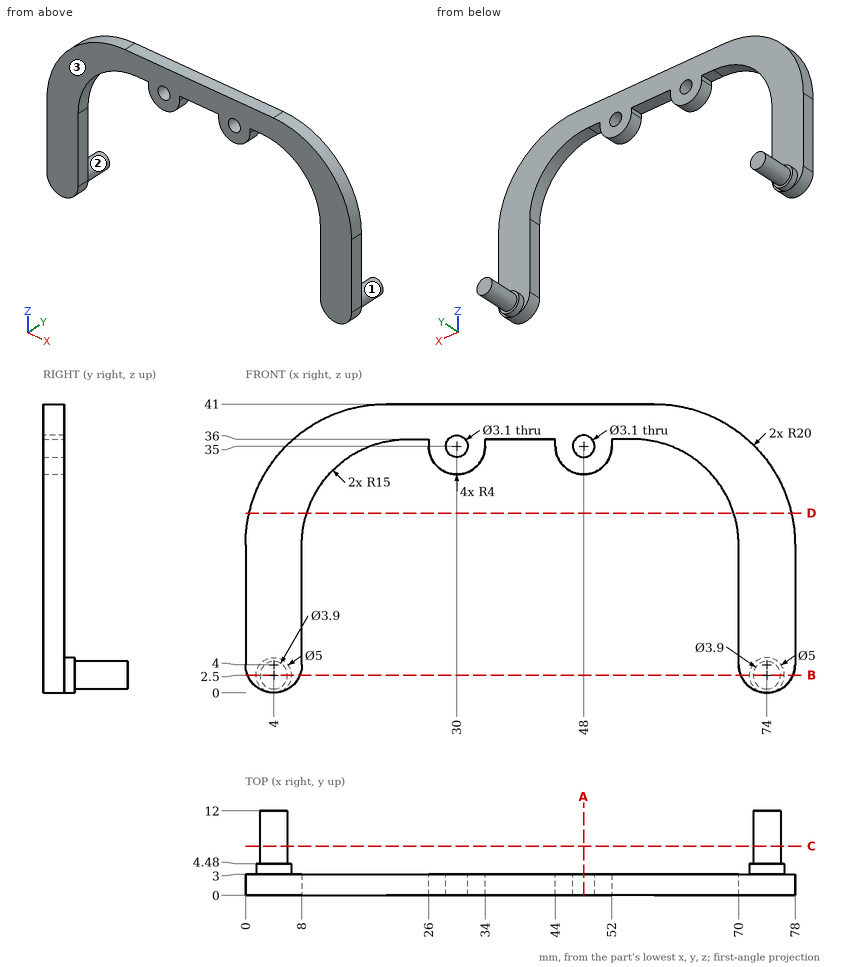
Can you work these out from the drawing? Everything is in mm from the part's minimum corner. Give positions to 0.01 mm unless a question says otherwise; leave off trailing zeros. Loops run counter-clockwise (first coordinate to the right, second up) from the corner with the lowest first, then second, coordinate; pieces in that order, holes last. Notation, with made-up numbers: (25.25, 59.5) - (34.25, 59.5) arc R24 cw to (34.25, 87.5) - close; hole circle Ø10 at (22, 47). An arc over 180 degrees is marked (long way). Use one line per item in the form item = value.
1. I want a section at D-D (z = 25.5). Please give me the cut outline in (x, y), and give its area (3 significant figures).
Response values:
outline = (0.51, 0) - (8.69, 0) - (8.69, 3) - (0.51, 3) - close; (69.31, 0) - (77.49, 0) - (77.49, 3) - (69.31, 3) - close
area = 49.1 mm²
2. I want a section at C-C (y = 7). Please give me the cut outline in (x, z), and give its area (3 significant figures).
Response values:
outline = circle Ø3.9 at (4, 2.5); circle Ø3.9 at (74, 2.5)
area = 23.9 mm²
3. I'm going to push flat-ended pins straight in: pin 1 Ø20.5 at (x, z) = (58, 28.5) entering from +Y; pin 2 Ø1.9 at (x, z) = (48, 35) entering from -Y; pin 3 Ø0.5 at (y, z) = (2, 35.5) entering from -X; pin 4 Ø0.8 at (y, z) = (1.5, 35.5) entering from +X. Where does each tip first touch, or does it pass through?
Response values:
pin_1 = 3
pin_2 = through
pin_3 = 5.97
pin_4 = 72.18
4. I need wall thicknesses on probe 1 along Z at (x, y) = (48, 1.35); probe 2 along Y at (x, z) = (59.5, 39); probe 3 along Z at (x, y) = (68, 2). Which ranges of each line are inside material? Lowest first, please.
Response values:
probe_1 = 31 to 33.45, 36.55 to 41
probe_2 = 0 to 3
probe_3 = 28.48 to 38.32
5. I want a section at A-A (x = 48). Please give me the cut outline in (y, z).
Response values:
outline = (0, 31) - (3, 31) - (3, 33.45) - (0, 33.45) - close; (0, 36.55) - (3, 36.55) - (3, 41) - (0, 41) - close
6. Thinking about a two-plate mould opening in X: for the marked faces 1, 2 and 3, which applies, released by +X, released by -X, zero draft, split by the parting line, or undercut?
Response values:
face_1 = undercut
face_2 = undercut
face_3 = zero draft
7. I want a section at B-B (z = 2.5). Please give me the cut outline in (x, y), and give its area (3 significant figures).
Response values:
outline = (0.29, 0) - (7.71, 0) - (7.71, 3) - (6.5, 3) - (6.5, 4.48) - (5.95, 4.48) - (5.95, 12) - (2.05, 12) - (2.05, 4.48) - (1.5, 4.48) - (1.5, 3) - (0.29, 3) - close; (70.29, 0) - (77.71, 0) - (77.71, 3) - (76.5, 3) - (76.5, 4.48) - (75.95, 4.48) - (75.95, 12) - (72.05, 12) - (72.05, 4.48) - (71.5, 4.48) - (71.5, 3) - (70.29, 3) - close
area = 118 mm²
